from build123d import *

# Parameters (mm, degrees)
SKETCH1_R           = 1.499947483
SKETCH1_W           = 3.194434014
SKETCH1_H           = 2.247005984
SKETCH1_W_2         = 3.194258538
SKETCH1_H_2         = 6.00021965
SKETCH1_W_3         = 14.9734805
SKETCH1_H_3         = 3.200030878
SKETCH1_W_4         = 9.982157856
SKETCH1_W_5         = 3.194239042
SKETCH1_H_4         = 4.3002681
SKETCH1_H_5         = 2.247064582
SKETCH1_H_6         = 4.300268101
SKETCH1_W_6         = 22.959156093
SKETCH1_H_7         = 12.400537771
BOSS_EXTRUDE1_DEPTH = 3.175


with BuildPart() as part:
    # Sketch1 → Boss-Extrude1 (new body)
    with BuildSketch(Plane(origin=(0, 0, 0), x_dir=(1, 0, 0), z_dir=(0, 1, 0))):
        with BuildLine():
            Line((-8.89863563, 14.616816531), (-8.898772113, -23.184447467))
            ThreePointArc((-8.898772113, -23.184447467), (-8.020049515, -25.305871479), (-5.898625504, -26.184594076))
            Line((-5.898625504, -26.184594076), (48.00009504, -26.184594076))
            ThreePointArc((48.00009504, -26.184594076), (50.117687721, -25.307458468), (50.994823329, -23.189865787))
            Line((50.994823329, -23.189865787), (50.994823329, 14.616811748))
            ThreePointArc((50.994823329, 14.616811748), (50.116118686, 16.738192414), (47.99473802, 17.616897057))
            Line((47.99473802, 17.616897057), (-5.904126705, 17.616897057))
            ThreePointArc((-5.904126705, 17.616897057), (-8.023535046, 16.737855239), (-8.89863563, 14.616816531))
        make_face()
        with Locations(Location((-4.406755257, 6.316598951, 0), (0, 0, 270))):
            Circle(SKETCH1_R, mode=Mode.SUBTRACT)
        with Locations(Location((30.531216432, -3.884174874, 0), (0, 0, 270))):
            Circle(SKETCH1_R, mode=Mode.SUBTRACT)
        with Locations(Location((46.602725133, 6.316403622, 0), (0, 0, 270))):
            Circle(SKETCH1_R, mode=Mode.SUBTRACT)
        with Locations(Location((30.531216431, -23.684709277, 0), (0, 0, 270))):
            Circle(SKETCH1_R, mode=Mode.SUBTRACT)
        with Locations((46.602666641, -2.060335363)):
            Rectangle(SKETCH1_W, SKETCH1_H, mode=Mode.SUBTRACT)
        with Locations((-4.506903026, -0.183533202)):
            Rectangle(SKETCH1_W_2, SKETCH1_H_2, mode=Mode.SUBTRACT)
        with Locations((36.121280984, 11.216808443)):
            Rectangle(SKETCH1_W_3, SKETCH1_H_3, mode=Mode.SUBTRACT)
        with Locations((3.678834136, 11.216808444)):
            Rectangle(SKETCH1_W_4, SKETCH1_H_3, mode=Mode.SUBTRACT)
        with Locations((-4.506717801, 13.66683384)):
            Rectangle(SKETCH1_W_5, SKETCH1_H_4, mode=Mode.SUBTRACT)
        with Locations((46.602666641, 1.692917368)):
            Rectangle(SKETCH1_W, SKETCH1_H_5, mode=Mode.SUBTRACT)
        with Locations((46.602666642, 13.666833838)):
            Rectangle(SKETCH1_W, SKETCH1_H_6, mode=Mode.SUBTRACT)
        with Locations((30.531148191, -14.184180414)):
            Rectangle(SKETCH1_W_6, SKETCH1_H_7, mode=Mode.SUBTRACT)
    extrude(amount=BOSS_EXTRUDE1_DEPTH)


solid = part.part
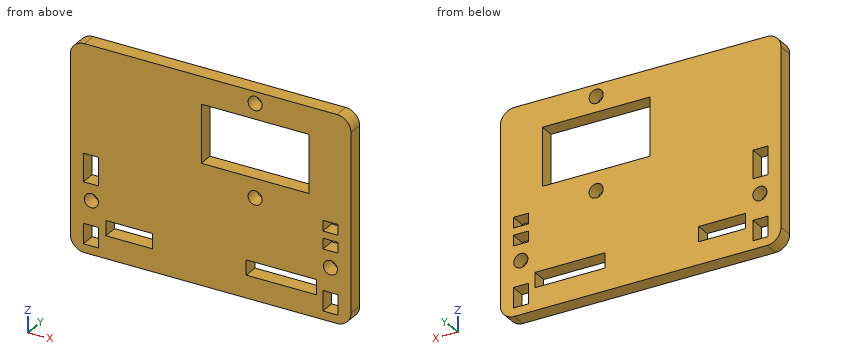
The model under review builds one solid part; all positions refer to its coordinate system, in mm. Round coordinates to 2 decimals unless told otherwise and drop trailing zeros. Loops run counter-clockwise (first coordinate to the right, second up) from the corner with the lowest first, then second, coordinate; pieces in that order, holes last. Notation, with made-up numbers: M 73.5,-10.5 L 131.5,-10.5 A13 cw 131.5,-4.5 Z; hole C 87.5,64.25 d1. An arc over 180 degrees is marked long. Answer as CSV lines item,"result". Start each with the question number.
Item 1: Consider section C-C (y = 0.95). State how many separate pieces and enclosed holes the cut face has, then the cut area to 3 significant figures.
Item 2: Consider section A-A (x = 2). Write out the cut boundary in (y, z) (3 decimals).
Item 3: Consider section B-B (z = 17.5). Write out the cut boundary in (x, y) (3 decimals).
Item 4: Wall thickness on line 1 (X direction, y = 1.5, z = -2.5); line 2 (X direction, y = 1, z = -11); line 3 (Z direction, x = 37, y = 2.6): over which ranges is each line inside the solid? List them lowest first. Write a range as [from, to].
Answer:
1,separate pieces,"1"
1,enclosed holes,"12"
1,area,"2,160 mm^2"
2,outline,"M 0,-17.617 L 3.175,-17.617 L 3.175,-12.817 L 0,-12.817 Z; M 0,-9.617 L 3.175,-9.617 L 3.175,26.185 L 0,26.185 Z"
3,outline,"M -8.899,0 L 19.052,0 L 19.052,3.175 L -8.899,3.175 Z; M 42.011,0 L 50.995,0 L 50.995,3.175 L 42.011,3.175 Z"
4,line 1,"x = [-8.9, -6.1], [-2.91, 45.01], [48.2, 50.99]"
4,line 2,"x = [-8.9, -1.31], [8.67, 28.63], [43.61, 50.99]"
4,line 3,"z = [-17.62, -12.82], [-9.62, 7.98], [20.38, 26.18]"
